```python
from build123d import *

# Parameters (mm, degrees)
EXTRUDE1_DEPTH = 90
EXTRUDE2_DEPTH = 85
EXTRUDE3_DEPTH = 91


with BuildPart() as part:
    # Sketch1 → Extrude1 (new body)
    with BuildSketch(Plane(origin=(0, 0, 0), x_dir=(1, 0, 0), z_dir=(0, 1, 0))):
        with BuildLine():
            Line((70, 0), (0, 0))
            Line((0, 0), (0, -70))
            ThreePointArc((0, -70), (49.497474683, -49.497474683), (70, 0))
        make_face()
    extrude(amount=EXTRUDE1_DEPTH)

    # Sketch2 → Extrude2 (add)
    with BuildSketch(Plane.ZY):
        Polygon((0, 70), (30, 70), (95, 15), (95, 0), (0, 0), align=None)
    extrude(amount=-EXTRUDE2_DEPTH)

    # Sketch3 → Extrude3 (cut, through all)
    with BuildSketch(Plane(origin=(0, 0, 0), x_dir=(1, 0, 0), z_dir=(0, 1, 0))):
        Polygon((85, -55), (50, -95), (85, -95), align=None)
    extrude(amount=EXTRUDE3_DEPTH, mode=Mode.SUBTRACT)


solid = part.part
```
Verification items for the finished model (mm, model axes). A direction names the side the tool comes from. Coordinates: 2 decimals unless noted, no trailing zeros. Write each loop counter-clockwise with the first axis right and the second up, starting at its lowest first coordinate (ties: lowest second). Pieces come first, ordered by that corner, then holes. Notation, with made-up numbers: M 12.5,55 L 57.5,55 A22 ccw 57.5,80 Z; hole C 46,52 d6. An arc over 180 degrees is marked long. One line per item, written item: value.
Item 1: Gauge pin test, flat ends, axial feed: pin 1 Ø4 at (x, y) = (62, 13) entering from +Z; pin 2 Ø1 at (x, z) = (39, 70) entering from +Y; pin 3 Ø8 at (y, z) = (80.5, 53.5) entering from +X; pin 4 Ø4 at (x, z) = (76, 70) entering from -Y. Record the tip position at first contact, or that the pin passes through.
Check sheet entries:
pin 1: stops at z = 83.57
pin 2: stops at y = 36.58
pin 3: stops at x = 49.49
pin 4: passes through
Item 2: Section check D-D, the plane y = 13.5. Record the boundary of the cut face in (x, z).
Check sheet entries:
outline: M 0,0 L 85,0 L 85,55 L 50,95 L 0,95 Z
Item 3: Scan lines: line 1 along X through (y, z) = (80.5, 49); line 2 along Y through (x, z) = (77, 4.5); line 3 along Z through (x, y) = (50, 17.5). Record each from-to range of solid material in increasing order.
Check sheet entries:
line 1: x = 0 to 49.99
line 2: y = 0 to 70
line 3: z = 0 to 92.05
Item 4: Access from +Z, -Z, +X, -X, +Y, -Y to the whole of each face (thin tool, end or side, straight path). Record for faces 1 (the flat face through (42, 0, 47)), 2 (the flat face through (42, 37, 69)).
Check sheet entries:
face 1: +Z, -Z, +X, -X, -Y
face 2: +Z, +X, +Y
Item 5: Section check B-B, the plane y = 76. Record the boundary of the cut face in (x, z).
Check sheet entries:
outline: M 0,0 L 70,0 A70 ccw 0,70 Z
Item 6: Section check A-A, the plane x = 16. Record the boundary of the cut face in (y, z), plus the area to 3 significant figures.
Check sheet entries:
outline: M 0,0 L 90,0 L 90,68.15 L 37.72,68.15 L 15,95 L 0,95 Z
area: 6,840 mm^2
Item 7: Section check C-C, the plane z = 59. Record the boundary of the cut face in (x, y).
Check sheet entries:
outline: M 0,0 L 81.5,0 L 81.5,45.46 L 37.67,45.46 L 37.67,90 L 0,90 Z
